Geometry: final body of the model. Coordinates: model frame, mm. Give positions to 0.01 mm unless a question says otherwise; leave off trailing zeros. Loops run counter-clockwise (first coordinate to the right, second up) from the corner with the lowest first, then second, coordinate; pieces in that order, holes last. Notation, with made-up numbers: (-8.5, 80) -> (45.5, 80) arc R32 cw to (45.5, 113) -> close; hole circle Ø6 at (47.5, 16). An arc over 180 degrees is marked (long way). Answer in a Markdown table with one row per item. Add a question column.
from build123d import *
from build123d import SkipClean  # not in build123d's __all__

# Parameters (mm, degrees)
F1_DEPTH = 10
F5_DEPTH = 10.001
F7_DEPTH = 10


with BuildPart() as f1:
    # F0 (on Top) → F1 (new body)
    with BuildSketch(Plane.XY):
        with BuildLine():
            Line((0, 240), (0, 0))
            Line((0, 0), (25, 0))
            Line((25, 0), (25, 250))
            ThreePointArc((25, 250), (17.6776695297, 267.6776695297), (0, 275))
            Line((0, 275), (0, 260))
            ThreePointArc((0, 260), (10, 250), (0, 240))
        make_face()
    extrude(amount=F1_DEPTH)

    # F2: F1 across face


with BuildPart() as f1_1:
    add(f1.part, clean=False)
    with SkipClean():  # cleaning this boolean's faces spoils the solid; the shape is the same uncleaned
        add(f1.part.mirror(Plane(origin=(0, 120, 5), x_dir=(0, -1, 0), z_dir=(-1, 0, 0))), clean=False)

    # F3: F1 across face


with BuildPart() as f1_2:
    add(f1_1.part, clean=False)
    add(f1_1.part.mirror(Plane(origin=(12.5, 0, 5), x_dir=(1, 0, 0), z_dir=(0, -1, 0))), clean=False)

    # F4 (on Top) → F5 (cut, through all)
    with BuildSketch(Plane.XY):
        Polygon((50, -200), (0, -250), (-50, -200), (-50, -344.7760872496), (50, -344.7760872496), align=None)
    extrude(amount=F5_DEPTH, mode=Mode.SUBTRACT)

    # F6 (on face) → F7 (join, through all)
    with BuildSketch(Plane.XY.offset(10)):
        Polygon((11.9149819948, -238.0850180052), (-11.0190114938, -238.9809885062), (0, -250), align=None)
    extrude(amount=-F7_DEPTH)


solid = f1_2.part
(1) Material intervals for line 1 along X through (y, z) = (250, 4.5); line 2 along Y through (x, z) = (0, 7.75); line 3 along Y through (x, z) = (-9, 2.75), sorted ascending. Write a range as from..to.
(2) Cut plane C-C on x = 18. Return the cut outline in (y, z).
(3) Cut plane B-B on x = -5. Return the cut outline in (y, z).
(4) Cut plane A-A on z = 8. Return the cut outline in (x, y).
(5) Pin query (flat end, axial travel): pin 1 Ø2 at (x, z) = (-9, 7.5) entering from +Y; pin 2 Ø16 at (x, y) = (0, 250) entering from -Z; pin 3 Ø6 at (x, z) = (-16, 2) entering from +Y; pin 4 Ø1 at (x, z) = (-1, 6.5) entering from +Y (3 decimals). Return the tip coordinate at first contact, or that it passes through.
(6) Draft query along Y for faces 1 (the cylindrical face through (-3, 259.54, 4.93)), 2 (the flat face through (0, 9, 0)), 3 (the flat face through (-12, -238, 5)). Return one class per face: +Y half, -Y half, draft (parallel to the pull), parting line (faces both ways), or undercut.
Answer list:
| question | item | result |
|---|---|---|
| 1 | line 1 | x = -25..-10, 10..25 |
| 1 | line 2 | y = -250..240, 260..275 |
| 1 | line 3 | y = -241..245.64, 254.36..273.32 |
| 2 | outline | (-232, 0) -> (267.35, 0) -> (267.35, 10) -> (-232, 10) -> close |
| 3 | outline | (-245, 0) -> (241.34, 0) -> (241.34, 10) -> (-245, 10) -> close; (258.66, 0) -> (274.49, 0) -> (274.49, 10) -> (258.66, 10) -> close |
| 4 | outline | (-25, -225) -> (0, -250) -> (25, -225) -> (25, 250) arc R25 ccw to (-25, 250) -> close; hole circle Ø20 at (0, 250) |
| 5 | pin 1 | stops at y = 273.69 |
| 5 | pin 2 | passes through |
| 5 | pin 3 | stops at y = 271.35 |
| 5 | pin 4 | stops at y = 274.995 |
| 6 | face 1 | undercut |
| 6 | face 2 | draft |
| 6 | face 3 | -Y half |
